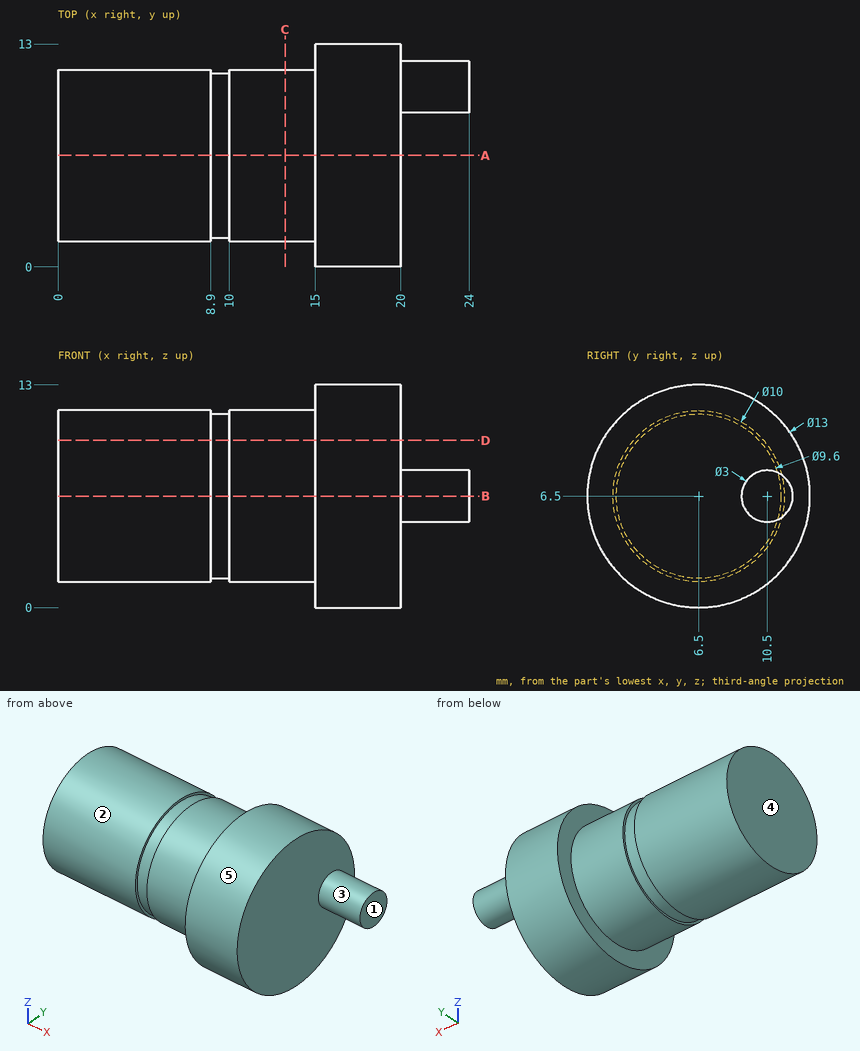
Geometry check sheet. Reference: drawing and pictorial views, mm from the part's lowest x, y, z. A direction names the side the tool comes from. Round coordinates to 2 decimals unless told otherwise and drop trailing zeros. Order: outer loops, then holes, each group sorted by start corner. A loop starts at its lowest first (then second) coordinate and runs counter-clockwise, first axis right, second up.
Q1. Cross-section at A-A, the plane y = 6.5. Enter the section's corners in (x, z), plus the area to 3 significant figures.
Filled sheet:
outline: (0, 1.5) - (8.9, 1.5) - (8.9, 1.7) - (10, 1.7) - (10, 1.5) - (15, 1.5) - (15, 0) - (20, 0) - (20, 13) - (15, 13) - (15, 11.5) - (10, 11.5) - (10, 11.3) - (8.9, 11.3) - (8.9, 11.5) - (0, 11.5) - close
area: 215 mm2
Q2. Scan lines: L1, parallel to Y at x = 13.75, z = 6.25; L2, parallel to X at y = 2.25, z = 7; L3, parallel to X at y = 2.75, z = 1.75. Record each from-to range of solid material in increasing order.
Filled sheet:
L1: y = 1.51 to 11.49
L2: x = 0 to 20
L3: x = 15 to 20
Q3. Cross-section at B-B, the plane z = 6.5. Enter the section's corners in (x, y), plus the area to 3 significant figures.
Filled sheet:
outline: (0, 1.5) - (8.9, 1.5) - (8.9, 1.7) - (10, 1.7) - (10, 1.5) - (15, 1.5) - (15, 0) - (20, 0) - (20, 9) - (24, 9) - (24, 12) - (20, 12) - (20, 13) - (15, 13) - (15, 11.5) - (10, 11.5) - (10, 11.3) - (8.9, 11.3) - (8.9, 11.5) - (0, 11.5) - close
area: 227 mm2
Q4. Set-up check for the marked faces 1, 2 and 3: record each of +Z, -Z, +X, -X, +Y, -Y from which the full face is reachable in a straight line by a thin tool's end or side.
Filled sheet:
face 1: +Z, -Z, +X, +Y, -Y
face 2: -X
face 3: +X
Q5. Cross-section at C-C, the plane x = 13.25. Enter the section's corners in (y, z).
Filled sheet:
outline: circle Ø10 at (6.5, 6.5)
Q6. Draft check along Y on the marked faces 4 and 5. Enter one of: pulls with the +Y half, pulls with the -Y half, needs draft (parallel to the pull), parting line crosses it, or undercut.
Filled sheet:
face 4: needs draft
face 5: parting line crosses it
Q7. Cross-section at D-D, the plane z = 9.75. Enter the section's corners in (x, y).
Filled sheet:
outline: (0, 2.7) - (8.9, 2.7) - (8.9, 2.97) - (10, 2.97) - (10, 2.7) - (15, 2.7) - (15, 0.87) - (20, 0.87) - (20, 12.13) - (15, 12.13) - (15, 10.3) - (10, 10.3) - (10, 10.03) - (8.9, 10.03) - (8.9, 10.3) - (0, 10.3) - close
Q8. Depth check by flat-ended pin: P1, Ø2, axis at x = 10, y = 4, coming from the -Z side; P2, Ø1, axis at x = 8.5, y = 3, coming from the +Z side; P3, Ø4, axis at x = 7, y = 5.5, coming from the -Z side. Enter the tip coordinate at first touch or a pass-through.
Filled sheet:
P1: stops at z = 1.73
P2: stops at z = 10.5
P3: stops at z = 1.5
